Verification items for the finished model (mm, model axes). A direction names the side the tool comes from. Give positions to 0.01 mm unless a question says otherwise; leave off trailing zeros. Loops run counter-clockwise (first coordinate to the right, second up) from the corner with the lowest first, then second, coordinate; pieces in that order, holes last. Notation, with made-up numbers: M 31,47.5 L 69,47.5 A18 ccw 69,61.5 Z; hole C -19.5,-2.5 d11. An arc over 180 degrees is marked long. Use a Markdown table: item, result.
from build123d import *

# Parameters (mm, degrees)
BOSS_EXTRUDE1_DEPTH = 5.24256
BOSS_EXTRUDE2_DEPTH = 4.03352
CHAMFER1_SIZE       = 3.2258
SKETCH3_R           = 3.2258
BOSS_EXTRUDE3_DEPTH = 0.80772
SKETCH4_R           = 2.42062
CUT_EXTRUDE1_DEPTH  = 2.42062


with BuildPart() as part:
    # Sketch1 → Boss-Extrude1 (new body)
    with BuildSketch(Plane.XY):
        Polygon((-8.87222, -7.86384), (8.87222, -7.86384), (8.87222, 7.86384), (4.03225, 7.86384), (4.03225, 4.63804), (5.64642, 4.63804), (5.64642, -2.21742), (-5.64642, -2.21742), (-5.64642, 4.63804), (-4.03225, 4.63804), (-4.03225, 7.86384), (-8.87222, 7.86384), align=None)
    extrude(amount=BOSS_EXTRUDE1_DEPTH)

    # Sketch2 → Boss-Extrude2 (add)
    with BuildSketch(Plane(origin=(0, 0, 0), x_dir=(-1, 0, 0), z_dir=(0, 0, -1))):
        with BuildLine():
            Line((-12.088220572, -2.21742), (12.088220572, -2.21742))
            ThreePointArc((12.088220572, -2.21742), (12.665396078, -2.456493922), (12.90447, -3.033669428))
            Line((12.90447, -3.033669428), (12.90447, -4.63804))
            ThreePointArc((12.90447, -4.63804), (11.959655055, -6.919025055), (9.67867, -7.86384))
            Line((9.67867, -7.86384), (-9.67867, -7.86384))
            ThreePointArc((-9.67867, -7.86384), (-11.959655055, -6.919025055), (-12.90447, -4.63804))
            Line((-12.90447, -4.63804), (-12.90447, -3.033669428))
            ThreePointArc((-12.90447, -3.033669428), (-12.665396078, -2.456493922), (-12.088220572, -2.21742))
        make_face()
    extrude(amount=BOSS_EXTRUDE2_DEPTH)

    # Chamfer1
    chamfer1_edges = [part.edges().sort_by_distance(p)[0] for p in [
        (0, -7.86384, 5.24256),
    ]]
    chamfer(chamfer1_edges, length=CHAMFER1_SIZE)

    # Sketch3 → Boss-Extrude3 (add)
    with BuildSketch(Plane(origin=(0, -2.21742, 0), x_dir=(1, 0, 0), z_dir=(0, 1, 0))):
        with Locations((0, -2.01676)):
            Circle(SKETCH3_R)
    extrude(amount=BOSS_EXTRUDE3_DEPTH)

    # Sketch4 → Cut-Extrude1 (cut)
    with BuildSketch(Plane(origin=(0, -1.4097, 0), x_dir=(1, 0, 0), z_dir=(0, 1, 0))):
        with Locations((0, -2.01676)):
            Circle(SKETCH4_R)
    extrude(amount=-CUT_EXTRUDE1_DEPTH, mode=Mode.SUBTRACT)


solid = part.part
(1) Gauge pin test, flat ends, axial feed: P1, Ø1.3, axis at x = -5, z = 4, coming from the -Y side; P2, Ø1, axis at x = 3, z = -1, coming from the +Y side; P3, Ø1.6, axis at y = 0, z = 2, coming from the +X side. Record the tip position at first contact, or that the pin passes through.
Results below:
| item | result |
|---|---|
| P1 | y = -6.53 |
| P2 | y = -2.22 |
| P3 | x = 8.87 |
(2) Material ranges on line 1 (X direction, y = 3, z = 2); line 2 (X direction, y = 5, z = 2); line 3 (X direction, y = -1.75, z = 3), recorded low to high.
Results below:
| item | result |
|---|---|
| line 1 | -8.87 to -5.65, 5.65 to 8.87 |
| line 2 | -8.87 to -4.03, 4.03 to 8.87 |
| line 3 | -8.87 to -5.65, -3.07 to -2.21, 2.21 to 3.07, 5.65 to 8.87 |
(3) Set-up check for faces 5 (the flat face through (-4.032, 6, 3)), 6 (the cylindrical face through (3.077, -1.819, 1.048)), 7 (the flat face through (5, 4.638, 3)): record each of +Z, -Z, +X, -X, +Y, -Y from which the full face is reachable in a straight line by a thin tool's end or side.
Results below:
| item | result |
|---|---|
| face 5 | +Z, -Z, +Y |
| face 6 | +Y |
| face 7 | +Z, -Z |
(4) Draft check along Y on faces 1 (the flat face through (0, -3.83, 2)), 2 (the flat face through (-7, 3, 0)), 3 (the flat face through (-5, 4.638, 3)), 4 (the flat face through (5.646, 1, 3)). Enter one of: +Y half, -Y half, draft (parallel to the pull), parting line (faces both ways), or undercut.
Results below:
| item | result |
|---|---|
| face 1 | +Y half |
| face 2 | draft |
| face 3 | undercut |
| face 4 | undercut |
(5) Cross-section at A-A on y = 1. Record the cut outline in (x, z), then the cut area to 3 significant figures.
Results below:
| item | result |
|---|---|
| outline | M -8.87,0 L -5.65,0 L -5.65,5.24 L -8.87,5.24 Z; M 5.65,0 L 8.87,0 L 8.87,5.24 L 5.65,5.24 Z |
| area | 33.8 mm^2 |
(6) Cross-section at D-D on z = 3.5. Record the cut outline in (x, y).
Results below:
| item | result |
|---|---|
| outline | M -8.87,-6.38 L 8.87,-6.38 L 8.87,7.86 L 4.03,7.86 L 4.03,4.64 L 5.65,4.64 L 5.65,-2.22 L 2.86,-2.22 L 2.86,-1.41 L 1.91,-1.41 L 1.91,-3.83 L -1.91,-3.83 L -1.91,-1.41 L -2.86,-1.41 L -2.86,-2.22 L -5.65,-2.22 L -5.65,4.64 L -4.03,4.64 L -4.03,7.86 L -8.87,7.86 Z |
(7) Cross-section at C-C on y = -6. Record the cut outline in (x, z), then the cut area to 3 significant figures.
Results below:
| item | result |
|---|---|
| outline | M -12.6,-4.03 L 12.6,-4.03 L 12.6,0 L 8.87,0 L 8.87,3.88 L -8.87,3.88 L -8.87,0 L -12.6,0 Z |
| area | 171 mm^2 |
(8) Cross-section at B-B on x = -7.75. Record the cut outline in (y, z).
Results below:
| item | result |
|---|---|
| outline | M -7.86,-4.03 L -2.22,-4.03 L -2.22,0 L 7.86,0 L 7.86,5.24 L -4.64,5.24 L -7.86,2.02 Z |
